Work out the finished part from the listing and answer in its coordinate system (mm). A direction names the side the tool comes from. Round coordinates to 2 decimals unless told otherwise and drop trailing zeros. Order: outer loops, then holes, each group sorted by start corner. A loop starts at its lowest first (then second) coordinate and runs counter-clockwise, first axis right, second up. Notation, with made-up numbers: (61, 38) -> (97, 38) arc R13 cw to (97, 57) -> close; hole circle Ø1 at (65.5, 85). An arc over 180 degrees is marked (long way). Use a Markdown table: item, result. Add a question column.
Item 1: A cutting plane is placed at C-C, the plane z = 2.75. Determine the outline of the cut face in (x, y).
Item 2: A cutting plane is placed at A-A, the plane x = 0. Determine the outline of the cut face in (y, z).
Item 3: Find the intervals of material crossed by L1, parallel to Y at x = 0, z = 2.8; L2, parallel to Y at x = 0, z = 0.8; L3, parallel to Z at x = -5, y = 1.25, in increasing order. Write a range as [from, to].
Item 4: Flat-ended cylindrical pins translate along their axes: P1, Ø1, axis at y = -2, z = 2, coming from the -X side; P2, Ø1.5, axis at x = 3.5, y = -3, coming from the +Z side; P3, Ø2, axis at y = -3, z = 2.5, coming from the -X side. Find the tip coordinate at first contact, or state that the pin passes through.
Item 5: A tool of negligible diameter and unlimited length cuts with its end or side. For faces 1 (the flat face through (2, -2, 0)), 2 (the cylindrical face through (-0.75, -5.7, 2.99)), from which of +Z, -Z, +X, -X, +Y, -Y can it reach the whole face along a straight path? Write none if from no direction.
Item 6: A cutting plane is placed at D-D, the plane y = 3. Determine the outline of the cut face in (x, z), plus the area to 3 significant figures.
Item 7: For a pull along X with two mould halves and no side action, classify faces 3 (the flat face through (-4.9, 3.3, 4)), 4 (the cylindrical face through (3.35, 6.43, 1.97)), 5 (the cylindrical face through (0, 2, 1)) as +X half, -X half, draft (parallel to the pull), parting line (faces both ways), or undercut.
Autodesk Fusion 360 part; units mm, degrees
sketch "Sketch1" plane through (0, 0, 0) normal (0, 0, 1) x (1, 0, 0)
  circle A0 centre (0, 0) radius 5.75
  circle A1 centre (0, 0) radius 7.25
  dimension "d1" = 11.5
  dimension "d9" = 1.5
extrude "Extrude1" add sketch "Sketch1" along normal blind 4
extrude "Extrude2" add sketch "Sketch1" along normal blind 2 contours A0
sketch "Sketch2" plane through (0, 0, 2) normal (0, 0, 1) x (-1, 0, 0)
  circle A0 centre (0, 0) radius 5.75
  circle A1 centre (0, 0) radius 2
  dimension "d6" = 4
extrude "Extrude3" cut sketch "Sketch2" against normal blind 5 contours A1
Reported:
| question | item | result |
|---|---|---|
| 1 | outline | circle Ø14.5 at (0, 0); hole circle Ø11.5 at (0, 0) |
| 2 | outline | (-7.25, 0) -> (-2, 0) -> (-2, 2) -> (-5.75, 2) -> (-5.75, 4) -> (-7.25, 4) -> close; (2, 0) -> (7.25, 0) -> (7.25, 4) -> (5.75, 4) -> (5.75, 2) -> (2, 2) -> close |
| 3 | L1 | [-7.25, -5.75], [5.75, 7.25] |
| 3 | L2 | [-7.25, -2], [2, 7.25] |
| 3 | L3 | [0, 2] |
| 4 | P1 | x = -7.09 |
| 4 | P2 | z = 2 |
| 4 | P3 | x = -6.97 |
| 5 | face 1 | -Z, +X, -X, +Y, -Y |
| 5 | face 2 | +Z |
| 6 | outline | (-6.6, 0) -> (6.6, 0) -> (6.6, 4) -> (4.91, 4) -> (4.91, 2) -> (-4.91, 2) -> (-4.91, 4) -> (-6.6, 4) -> close |
| 6 | area | 33.2 mm² |
| 7 | face 3 | draft |
| 7 | face 4 | parting line |
| 7 | face 5 | undercut |
